Geometry: final body of the model. Coordinates: model frame, mm. A direction names the side the tool comes from. Round coordinates to 2 decimals unless told otherwise and drop trailing zeros. Order: outer loops, then holes, each group sorted by start corner. A loop starts at its lowest first (then second) coordinate and runs counter-clockwise, first axis right, second up. Notation, with made-up numbers: M 28.25,64.5 L 56.25,64.5 A22 ccw 56.25,80.5 Z; hole C 9.5,-37 d2. An arc over 180 degrees is marked long. Put each result on its own line as item: value. Start each with the question number.
1) Draft query along Y for faces 1 (the cylindrical face through (3, -5, 4)), 2 (the flat face through (2.2, 30, -3.3)), 3 (the conical face through (-2.363, 0.621, -4.544)). Return one class per face: pulls with the +Y half, pulls with the -Y half, needs draft (parallel to the pull), parting line crosses it, or undercut.
2) Section B-B, the plane x = 0. Return loops of the section in (y, z), then the cut area to 4 significant figures.
3) Material intervals for probe 1 along Z at (x, y) = (0, 17); probe 2 along Z at (x, y) = (-0.25, -0.5); probe 3 along X at (y, z) = (24.5, 0), sorted ascending. Write a range as [from, to].
4) First-contact query: P1, Ø5.5, axis at x = 0, z = 0, coming from the +Y side; P2, Ø1, axis at x = 4, z = -5, coming from the -Y side; P3, Ø8, axis at y = 22.5, z = -5.5, coming from the -X side. Flat tips, straight axial feed; report the tip coordinate or a pass-through.
5) Section A-A, the plane z = 0. Return loops of the section in (x, y).
6) Section C-C, the plane y = -2. Return loops of the section in (x, z), then the cut area to 3 significant figures.
7) Section D-D, the plane y = 2. Return loops of the section in (x, z).
8) Access query for faces 4 (the cylindrical face through (7.493, 10.098, 0.33)), 5 (the cylindrical face through (3, 25, 4)). Directions: +Z, -Z, +X, -X, +Y, -Y. A direction counts if a zero-diameter tool reaches every point of the face in a straight line with its end or side. Return the directions, or none.
from build123d import *

# Parameters (mm, degrees)
F0_R         = 5
F0_R_2       = 3.5
F1_DEPTH     = 10
F2_R         = 7.5
F2_R_2       = 5
F2_R_3       = 3.5
F3_DEPTH     = 10
F5_S5_R      = 5
F5_T6_DEPTH  = 12
F5_S11_R     = 5
F5_T12_DEPTH = 12


# Not quite as in the source:
# - a fillet or chamfer that OpenCascade refuses, or shapes differently, is made with other operations: its cross-section is extruded or revolved along the edge and cut away or added


with BuildPart() as f1:
    # F0 (on Front) → F1 (new body)
    with BuildSketch(Plane.XZ):
        Circle(F0_R)
        Circle(F0_R_2, mode=Mode.SUBTRACT)
    extrude(amount=F1_DEPTH)

    # F2 (on face) → F3 (join)
    with BuildSketch(Plane(origin=(0, 0, 0), x_dir=(-1, 0, 0), z_dir=(0, 1, 0))):
        Circle(F2_R)
        Circle(F2_R_2, mode=Mode.SUBTRACT)
        Circle(F2_R_2)
        Circle(F2_R_3, mode=Mode.SUBTRACT)
    extrude(amount=F3_DEPTH)

    # F4: F1 across face


with BuildPart() as f1_1:
    add(f1.part)
    add(f1.part.mirror(Plane(origin=(0, 10, 0), x_dir=(-1, 0, 0), z_dir=(0, 1, 0))))

    # F5: chamfer of 3 on 2 edges, made by hand


with BuildPart() as f5_tool2:
    # F5_s3 → F5_t4 (revolve)
    with BuildSketch(Plane.XY):
        Polygon((-4.5, 20), (-7.5, 17), (-7.5, 20), align=None)
    revolve(axis=Axis((0, 20, 0), (0, 1, 0)))

    # F5_s5 → F5_t6 (cut, symmetric)
    with BuildSketch(Plane.XZ.offset(-18.5)):
        Circle(F5_S5_R)
    extrude(amount=F5_T6_DEPTH, both=True, mode=Mode.SUBTRACT)


with BuildPart() as f1_2:
    add(f1_1.part)

    # F5_t1: cut F5_tool2
    add(f5_tool2.part, mode=Mode.SUBTRACT)


with BuildPart() as f5_tool8:
    # F5_s9 → F5_t10 (revolve)
    with BuildSketch(Plane.XY):
        Polygon((-7.5, 3), (-4.5, 0), (-7.5, 0), align=None)
    revolve(axis=Axis((0, 0, 0), (0, 1, 0)))

    # F5_s11 → F5_t12 (cut, symmetric)
    with BuildSketch(Plane.XZ.offset(-1.5)):
        Circle(F5_S11_R)
    extrude(amount=F5_T12_DEPTH, both=True, mode=Mode.SUBTRACT)


with BuildPart() as f1_3:
    add(f1_2.part)

    # F5_t7: cut F5_tool8
    add(f5_tool8.part, mode=Mode.SUBTRACT)


solid = f1_3.part
Result sheet:
1. face 1: needs draft
1. face 2: pulls with the +Y half
1. face 3: pulls with the -Y half
2. outline: M -10,-5 L 0.5,-5 L 3,-7.5 L 17,-7.5 L 19.5,-5 L 30,-5 L 30,-3.5 L -10,-3.5 Z; M -10,3.5 L 30,3.5 L 30,5 L 19.5,5 L 17,7.5 L 3,7.5 L 0.5,5 L -10,5 Z
2. area: 202.5 mm2
3. probe 1: z = [-7.5, -3.5], [3.5, 7.5]
3. probe 2: z = [-4.99, -3.49], [3.49, 4.99]
3. probe 3: x = [-5, -3.5], [3.5, 5]
4. P1: passes through
4. P2: stops at y = 1.4
4. P3: stops at x = -4.77
5. outline: M -7.5,3 L -5,0.5 L -5,-10 L -3.5,-10 L -3.5,30 L -5,30 L -5,19.5 L -7.5,17 Z; M 3.5,-10 L 5,-10 L 5,0.5 L 7.5,3 L 7.5,17 L 5,19.5 L 5,30 L 3.5,30 Z
6. outline: C 0,0 d10; hole C 0,0 d7
6. area: 40.1 mm2
7. outline: C 0,0 d13; hole C 0,0 d7
8. face 4: +Y, -Y
8. face 5: +Y
